Can you work these out from the model? Positions are in its coordinate system, mm. Give positions to 0.01 mm unless a question says otherwise; leave off trailing zeros. Loops run counter-clockwise (first coordinate to the right, second up) from the corner with the lowest first, then second, coordinate; pieces in that order, holes last. Notation, with made-up numbers: M -18.75,83.25 L -12.75,83.25 A23 cw -12.75,121.25 Z; hole C -9.5,78.25 d6. An arc over 180 degrees is marked long. Use CSV: the item, a comma, the result in double quotes.
from build123d import *

# Parameters (mm, degrees)
ESQUISSE1_W                     = 355.6
ESQUISSE1_H                     = 50.8
BOSS_EXTRU_1_DEPTH              = 6.35
ESQUISSE2_W                     = 6.35
ESQUISSE2_H                     = 10.16
ENL_V_MAT_EXTRU_1_DEPTH         = 180.717340566
R_P_TITION_LIN_AIRE1_COUNT      = 2
R_P_TITION_LIN_AIRE1_PITCH      = 20.32
R_P_TITION_LIN_AIRE1_COUNT_DIR2 = 2
R_P_TITION_LIN_AIRE1_PITCH_DIR2 = 349.25
ESQUISSE3_W                     = 25.4
ESQUISSE3_H                     = 6.35
BOSS_EXTRU_2_DEPTH              = 6.35
R_P_TITION_LIN_AIRE2_COUNT      = 7
R_P_TITION_LIN_AIRE2_PITCH      = 50.8


with BuildPart() as part:
    # Esquisse1 → Boss.-Extru.1 (new body)
    with BuildSketch(Plane.XY):
        Rectangle(ESQUISSE1_W, ESQUISSE1_H)
    extrude(amount=BOSS_EXTRU_1_DEPTH)

    # Esquisse2 → Enlèv. mat.-Extru.1 (cut, through all)
    with BuildSketch(Plane.XY.offset(6.35)):
        with Locations((-174.625, -10.16)):
            Rectangle(ESQUISSE2_W, ESQUISSE2_H)
    enl_v_mat_extru_1 = extrude(amount=-ENL_V_MAT_EXTRU_1_DEPTH, mode=Mode.SUBTRACT)

    # Répétition linéaire1: Enl_v. mat.-Extru.1 2 × 2
    with Locations(*[(j * R_P_TITION_LIN_AIRE1_PITCH_DIR2, i * R_P_TITION_LIN_AIRE1_PITCH, 0) for i in range(R_P_TITION_LIN_AIRE1_COUNT) for j in range(R_P_TITION_LIN_AIRE1_COUNT_DIR2) if (i, j) != (0, 0)]):
        add(enl_v_mat_extru_1, mode=Mode.SUBTRACT)

    # Esquisse3 → Boss.-Extru.2 (add)
    with BuildSketch(Plane.XY.offset(6.35)):
        with Locations((-152.4, -28.575)):
            Rectangle(ESQUISSE3_W, ESQUISSE3_H)
    boss_extru_2 = extrude(amount=-BOSS_EXTRU_2_DEPTH)

    # Répétition linéaire2: Boss.-Extru.2 ×7
    with Locations(*[(i * R_P_TITION_LIN_AIRE2_PITCH, 0, 0) for i in range(1, R_P_TITION_LIN_AIRE2_COUNT)]):
        add(boss_extru_2)


solid = part.part
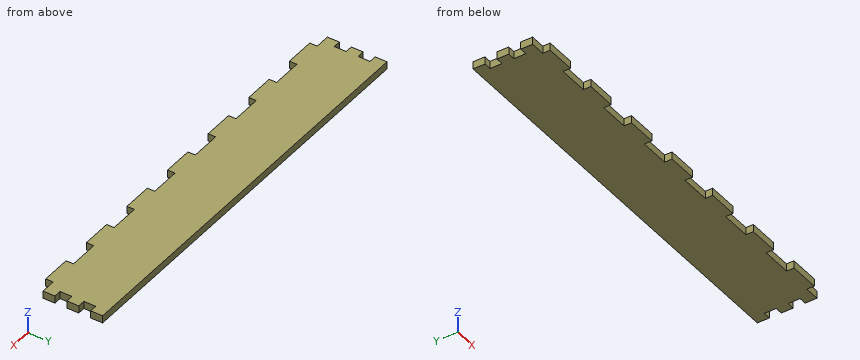
Q1. I want a section at A-A, the plane y = 10. Please give me the cut outline in (x, z).
Model answer:
outline,"M -171.45,0 L 171.45,0 L 171.45,6.35 L -171.45,6.35 Z"
Q2. I'm going to push flat-ended pins straight in: P1, Ø1.9, axis at y = -28.5, z = 2.5, coming from the +X side; P2, Ø1.9, axis at x = 122, z = 4.5, coming from the -Y side; P3, Ø1.5, axis at x = 123.5, y = -3, coming from the -Z side; P4, Ø3, axis at y = -28.5, z = 4.5, coming from the -X side. Where does each tip first touch, or does it pass through?
Model answer:
P1,"x = 165.1"
P2,"y = -25.4"
P3,"z = 0"
P4,"x = -165.1"
Q3. Please list where these lines run through material, in increasing order: L1, parallel to X at y = -12.5, z = 2.5; L2, parallel to Y at x = -21.5, z = 1.75. Write a range as from..to.
Model answer:
L1,"-171.45..171.45"
L2,"-25.4..25.4"
Q4. I want a section at B-B, the plane x = 83.5. Please give me the cut outline in (y, z).
Model answer:
outline,"M -25.4,0 L 25.4,0 L 25.4,6.35 L -25.4,6.35 Z"
